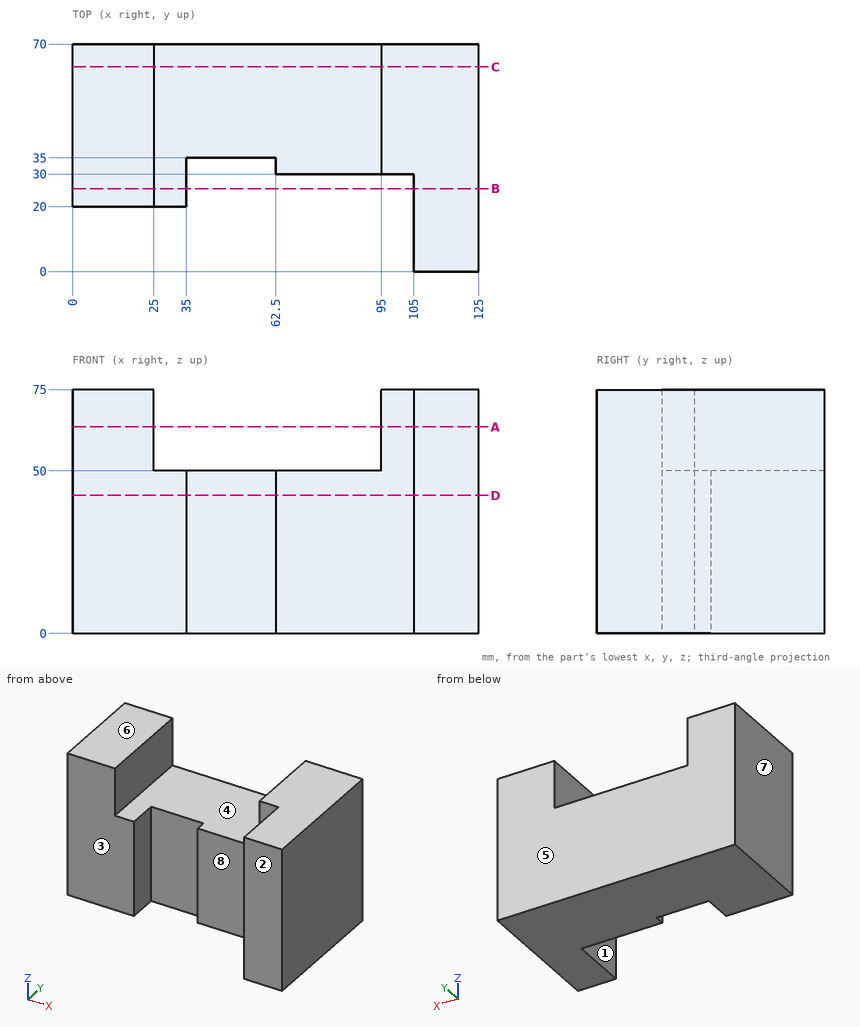
For this review, use the dimensioned drawing (mm, ordinates from the lowest corner) and the shaded views. A direction names the side the tool comes from. Give positions to 0.01 mm unless a question says otherwise; leave off trailing zeros. Write each loop counter-clockwise with the first axis right and the second up, starting at its lowest first coordinate (ties: lowest second). Pieces come first, ordered by that corner, then holes.
(1) The part is to be moulded in two halves that separate along X. For the marked faces 6, 7 and 8, say which applies: released by +X, released by -X, zero draft, split by the parting line, or undercut.
(2) Consider section C-C, the plane y = 63. Give the boundary of the cut face in (x, z).
(3) Consider section B-B, the plane y = 25.5. Give the boundary of the cut face in (x, z).
(4) To check wall thickness, follow L1, parallel to X at y = 41, z = 50.5; L2, parallel to X at y = 25, z = 19; L3, parallel to Y at x = 6.5, z = 47. State the ranges of each line that lie inside material, in increasing order.
(5) Consider section D-D, the plane z = 42.5. Give the boundary of the cut face in (x, y), and give its area (3 significant figures).
(6) For P1, Ø9, axis at y = 13.5, z = 24, coming from the -X side; P2, Ø3, axis at x = 98.5, z = 59, coming from the -Y side; P3, Ø10.5, axis at x = 25.5, z = 33, coming from the -Y side, all flat-tipped, find the tip position at first contact; note any pin that passes through.
(7) Consider section A-A, the plane z = 63.5. Give the boundary of the cut face in (x, y), and give its area (3 significant figures).
(8) Tool access review of the marked faces 1, 2, 3, 4 and 5: name each direction out of +Z, -Z, +X, -X, +Y, -Y from which nothing blocks a thin tool from reaching the whole face with its end or side.
Returned:
1. face 6: zero draft
1. face 7: released by -X
1. face 8: undercut
2. outline: (0, 0) - (125, 0) - (125, 75) - (95, 75) - (95, 50) - (25, 50) - (25, 75) - (0, 75) - close
3. outline: (0, 0) - (35, 0) - (35, 50) - (25, 50) - (25, 75) - (0, 75) - close; (105, 0) - (125, 0) - (125, 75) - (105, 75) - close
4. L1: x = 0 to 25, 95 to 125
4. L2: x = 0 to 35, 105 to 125
4. L3: y = 20 to 70
5. outline: (0, 20) - (35, 20) - (35, 35) - (62.5, 35) - (62.5, 30) - (105, 30) - (105, 0) - (125, 0) - (125, 70) - (0, 70) - close
5. area: 5,810 mm2
6. P1: stops at x = 105
6. P2: stops at y = 30
6. P3: stops at y = 20
7. outline: (0, 20) - (25, 20) - (25, 70) - (0, 70) - close; (95, 30) - (105, 30) - (105, 0) - (125, 0) - (125, 70) - (95, 70) - close
7. area: 3,050 mm2
8. face 1: +Z, -Z, -Y
8. face 2: +Z, -Z, +X, -X, -Y
8. face 3: +Z, -Z, -X, -Y
8. face 4: +Z, +Y, -Y
8. face 5: +Z, -Z, +X, -X, +Y
